Autodesk Inventor part; units mm, degrees
ref_plane "YZ Plane" through (0, 0, 0) normal (1, 0, 0) x (0, 1, 0)
ref_plane "XZ Plane" through (0, 0, 0) normal (0, 1, 0) x (-1, 0, 0)
ref_plane "XY Plane" through (0, 0, 0) normal (0, 0, 1) x (1, 0, 0)
sketch "Sketch1" plane through (0, 0, 0) normal (0, 1, 0) x (-1, 0, 0)
  line L0 (0, 0) -> (200, 0)
  line L1 (200, 0) -> (200, -190)
  line L2 (200, -190) -> (0, -190)
  line L3 (0, -190) -> (0, 0)
  dimension "d0" = 200
  dimension "d1" = 190
extrude "Extrusion1" add sketch "Sketch1" along normal blind 9
sketch "Sketch10" plane through (0, 9, 0) normal (0, 1, 0) x (1, 0, 0)
  line L0 (0, 190) -> (-200, 190)
  line L1 (-200, 190) -> (-200, 0)
  line L2 (-200, 0) -> (0, 0)
  line L3 (0, 0) -> (0, 190)
  circle A0 centre (-100, 95) radius 15
  dimension "d27" = 30
extrude "Extrusion10" cut sketch "Sketch10" against normal blind 9 contours A0
sketch "Sketch14" plane through (0, 9, 0) normal (0, 1, 0) x (1, 0, 0)
  circle A0 centre (-100, 95) radius 15
  line L0 (0, 190) -> (-200, 190)
  line L1 (-200, 190) -> (-200, 0)
  line L2 (-200, 0) -> (0, 0)
  line L3 (0, 0) -> (0, 190)
  line L4 (-200, 190) -> (-200, 0)
  line L5 (-200, 190) -> (0, 190)
  line L6 (0, 190) -> (0, 181)
  line L7 (0, 181) -> (-200, 181)
  line L8 (-200, 181) -> (-200, 190)
  line L9 (-200, 0) -> (0, 0)
  line L10 (-200, 181) -> (-191, 181)
  line L11 (-191, 181) -> (-191, 0)
  line L12 (-191, 0) -> (-200, 0)
  line L13 (-200, 0) -> (-200, 181)
  line L14 (0, 0) -> (0, 190)
  line L15 (-191, 0) -> (0, 0)
  line L16 (0, 0) -> (0, 9)
  line L17 (0, 9) -> (-191, 9)
  line L18 (-191, 9) -> (-191, 0)
  circle A1 centre (-10, 4.5) radius 1.5
  circle A2 centre (-100, 4.5) radius 1.5
  circle A3 centre (-181, 4.5) radius 1.5
  line L19 (-245.0017, 95) -> (56.9583, 95)
  circle A4 centre (-10, 185.5) radius 1.5
  circle A5 centre (-100, 185.5) radius 1.5
  circle A6 centre (-181, 185.5) radius 1.5
  circle A7 centre (-195.5, 95) radius 1.5
  circle A8 centre (-195.5, 171) radius 1.5
  circle A9 centre (-195.5, 19) radius 1.5
  dimension "d47" = 9
  dimension "d48" = 9
  dimension "d49" = 9
  dimension "d50" = 3
  dimension "d51" = 3
  dimension "d52" = 3
  dimension "d55" = 3
  dimension "d56" = 3
  dimension "d57" = 3
extrude "Extrusion14" cut sketch "Sketch14" against normal blind 10 contours A1 | A2 | A3 | A4 | A5 | A6
extrude "Extrusion15" cut sketch "Sketch14" against normal blind 10 contours A7 L19 | L19 A7 | A8 | A9
properties part number "BaseEncima_3DPrint"
Design review of the part built by this model. Coordinates are the model's own, in mm. Coordinates: 2 decimals unless noted, no trailing zeros. Order: outer loops, then holes, each group sorted by start corner. A loop starts at its lowest first (then second) coordinate and runs counter-clockwise, first axis right, second up.
Item 1: For pin 1 Ø5 at (x, z) = (-10, -4.5) entering from -Y, flat-tipped, find the tip position at first contact; note if it passes through.
Item 2: For line 1 (X direction, y = 2.5, z = -95); line 2 (X direction, y = 5.75, z = -4.5); line 3 (X direction, y = 8.75, z = -104.5), list the stretches that pass through material, from the lowest coordinate up.
Item 3: Take a section at B-B, the plane z = -84.5. Write out the cut boundary in (x, y).
Item 4: Take a section at A-A, the plane y = 3.75. Count the separate pieces of the cut face and the enclosed holes in it, then the cut area to 3 significant figures.
Item 5: The part is to be moulded in two halves that separate along Z. For faces 1 (the cylindrical face through (-103.252, 4.563, -80.357)), 2 (the flat face through (-101, 4, -190)), 3 (the flat face through (-99, 4, 0)), 4 (the flat face through (-99, 0, -115)), say which applies: pulls with the +Z half, pulls with the -Z half, needs draft (parallel to the pull), parting line crosses it, or undercut.
The answers:
1. pin 1: stops at y = 0
2. line 1: x = -200 to -197, -194 to -115, -85 to 0
2. line 2: x = -200 to -182.5, -179.5 to -101.5, -98.5 to -11.5, -8.5 to 0
2. line 3: x = -200 to -111.61, -88.39 to 0
3. outline: (-200, 0) - (-110.71, 0) - (-110.71, 9) - (-200, 9) - close; (-89.29, 0) - (0, 0) - (0, 9) - (-89.29, 9) - close
4. separate pieces: 1
4. enclosed holes: 10
4. area: 37,200 mm2
5. face 1: undercut
5. face 2: pulls with the -Z half
5. face 3: pulls with the +Z half
5. face 4: needs draft
